Can you work these out from the drawing? Everything is in mm from the part's minimum corner. A direction names the side the tool comes from. Give positions to 0.01 mm unless a question says otherwise; leave off trailing zeros. Loops run counter-clockwise (first coordinate to the right, second up) from the corner with the lowest first, then second, coordinate; pieces in that order, holes last. Notation, with made-up numbers: (-7.5, 58.5) - (-2.5, 58.5) arc R25 ccw to (-2.5, 85.5) - close; hole circle Ø8 at (12, 44.25). An arc over 180 degrees is marked (long way). Answer in a Markdown table with one row per item. Add a question column.
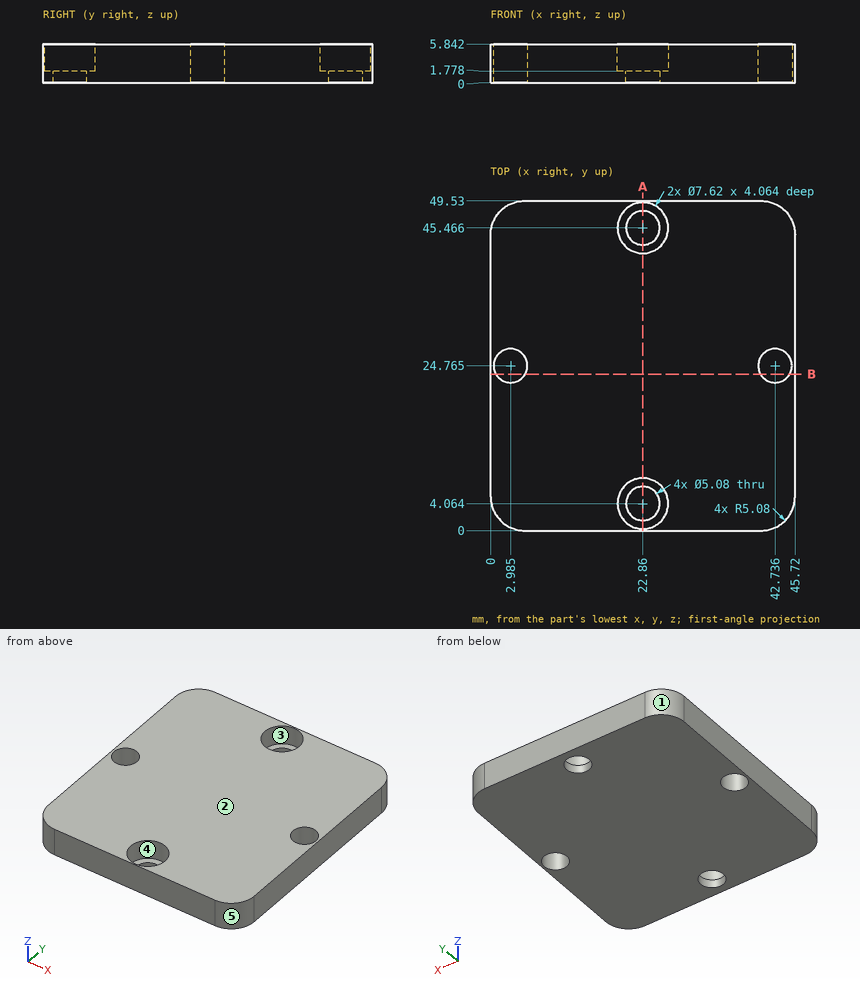
(1) We'd pull the mould along X, two halves only. Please class the marked faces 1, 2 and 3: pulls with the +X half, pulls with the -X half, needs draft (parallel to the pull), parting line crosses it, or undercut.
(2) I want a section at A-A on x = 22.86. State how many separate pieces and enclosed holes the cut face has, then the cut area to 3 significant figures.
(3) I want a section at B-B on y = 23.5. Please give me the cut outline in (x, z).
(4) Please list where these lines run through material, in increasing order: line 1 (Y direction, x = 22.86, z = 0.7) (1 decimal); line 2 (Y direction, x = 25, z = 1.4) (1 decimal); line 3 (X direction, y = 26, z = 4.25) (1 decimal).
(5) For pin 1 Ø4 at (x, y) = (22.5, 45) entering from +Z; pin 2 Ø4 at (x, y) = (42.74, 24.76) entering from +Z, each with a flat end and sliding along its axis, tell me the tip position at first contact or that it passes through.
(6) On a 3-axis mill with a long thin cutter (end or side, diameter ignored), from which of +Z, -Z, +X, -X, +Y, -Y can I reach the whole of each face in a straight line? I mean the marked faces 4 and 5. Say none if no direction works.
Reported:
| question | item | result |
|---|---|---|
| 1 | face 1 | pulls with the -X half |
| 1 | face 2 | needs draft |
| 1 | face 3 | undercut |
| 2 | separate pieces | 3 |
| 2 | enclosed holes | 0 |
| 2 | area | 209 mm² |
| 3 | outline | (0, 0) - (0.78, 0) - (0.78, 5.84) - (0, 5.84) - close; (5.19, 0) - (40.53, 0) - (40.53, 5.84) - (5.19, 5.84) - close; (44.94, 0) - (45.72, 0) - (45.72, 5.84) - (44.94, 5.84) - close |
| 4 | line 1 | 0 to 1.5, 6.6 to 42.9, 48 to 49.5 |
| 4 | line 2 | 0 to 2.7, 5.4 to 44.1, 46.8 to 49.5 |
| 4 | line 3 | 0 to 0.8, 5.2 to 40.5, 45 to 45.7 |
| 5 | pin 1 | z = 1.78 |
| 5 | pin 2 | through |
| 6 | face 4 | +Z |
| 6 | face 5 | +Z, -Z, +X, -Y |
